The listing builds one solid part. Answer for the finished solid, in the listing's coordinates (mm). Face numbers are marked on the shaded views. Round coordinates to 2 decimals unless told otherwise and drop trailing zeros. Write each loop counter-clockwise with the first axis right and the second up, starting at its lowest first coordinate (ties: lowest second). Pieces come first, ordered by that corner, then holes. Notation, with made-up numbers: (-20.75, -10.75) - (-3.75, -10.75) arc R26 ccw to (-3.75, 11.25) - close; hole circle Ø11 at (-20, -37.5). An arc over 180 degrees is marked (long way). Use a Markdown table: item, result. Add a question column.
1) A cutting plane is placed at C-C (y = 24.5). Give the vertices of the cut face in (x, z) (3 decimals).
2) Each of these flat-tipped pins is pushed along its axis until it touches: P1, Ø5, axis at y = 7, z = 12.5, coming from the -X side; P2, Ø4.5, axis at x = -33.23, y = -33.23, coming from the -Z side; P3, Ø3, axis at x = -1.5, y = 22.5, coming from the +Z side; P4, Ø1.5, axis at x = -4, z = 3.5, coming from the +Y side. Where does it stop, or does it pass through?
3) A cutting plane is placed at A-A (z = 2.25). State how many separate pieces and enclosed holes the cut face has, then the cut area to 3 significant figures.
4) A cutting plane is placed at D-D (z = 9.75). Give the vertices of the cut face in (x, y), then the cut area to 3 significant figures.
5) Determine the mould class of the marked faces 1, 2, 3 and 4 for opening direction Y: +Y half, -Y half, draft (parallel to the pull), parting line (faces both ways), or undercut.
6) Find the intervals of material crossed by probe 1 along Y at (x, z) = (0, 21); probe 2 along Y at (x, z) = (-3, 18); probe 3 along Y at (x, z) = (-1, 10), in increasing order. Write a range as from..to.
7) A cutting plane is placed at B-B (x = -7.5). Give the vertices of the cut face in (y, z), then the cut area to 3 significant figures.
```python
from build123d import *

# Parameters (mm, degrees)
SKETCH1_R                       = 35
SKETCH1_R_2                     = 26
BOSS_EXTRUDE1_DEPTH             = 5
F_3_0MM_DOWEL_HOLE1_D           = 3
F_3_0MM_DOWEL_HOLE1_CSINK_D     = 3.05
F_3_0MM_DOWEL_HOLE1_CSINK_ANGLE = 90
SKETCH5_R                       = 40
SKETCH5_R_2                     = 35
BOSS_EXTRUDE2_DEPTH             = 22
BOSS_EXTRUDE3_START             = -5
SKETCH6_R                       = 52
SKETCH6_R_2                     = 35
BOSS_EXTRUDE3_DEPTH             = 5
F_4_0MM_DOWEL_HOLE2_D           = 4
F_4_0MM_DOWEL_HOLE2_CSINK_D     = 4.05
F_4_0MM_DOWEL_HOLE2_CSINK_ANGLE = 90
CUT_EXTRUDE1_DEPTH              = 3


with BuildPart() as part:
    # Sketch1 → Boss-Extrude1 (new body)
    with BuildSketch(Plane.XY):
        Circle(SKETCH1_R)
        Circle(SKETCH1_R_2, mode=Mode.SUBTRACT)
    extrude(amount=BOSS_EXTRUDE1_DEPTH)

    # Ø3.0mm Dowel Hole1 (through all)
    with Locations(Plane(origin=(0, 0, 0), x_dir=(-1, 0, 0), z_dir=(0, 0, -1))):
        with Locations((21.213203436, 21.213203436), (0, 30), (-21.213203436, 21.213203436), (-30, 0), (-21.213203436, -21.213203436), (0, -30), (21.213203436, -21.213203436), (30, 0)):
            CounterSinkHole(F_3_0MM_DOWEL_HOLE1_D / 2, F_3_0MM_DOWEL_HOLE1_CSINK_D / 2, counter_sink_angle=F_3_0MM_DOWEL_HOLE1_CSINK_ANGLE)

    # Sketch5 → Boss-Extrude2 (add)
    with BuildSketch(Plane(origin=(0, 0, 0), x_dir=(-1, 0, 0), z_dir=(0, 0, -1))):
        Circle(SKETCH5_R)
        Circle(SKETCH5_R_2, mode=Mode.SUBTRACT)
    extrude(amount=-BOSS_EXTRUDE2_DEPTH)

    # Sketch6 → Boss-Extrude3 (add)
    with BuildSketch(Plane.XY.offset(22).offset(BOSS_EXTRUDE3_START)):
        Circle(SKETCH6_R)
        with Locations(Location((0, 0, 0), (0, 0, 180))):
            Circle(SKETCH6_R_2, mode=Mode.SUBTRACT)
    extrude(amount=BOSS_EXTRUDE3_DEPTH)

    # Ø4.0mm Dowel Hole2 (through all)
    with Locations(Plane.XY.offset(22)):
        with Locations((0, 47), (-33.234018716, 33.234018716), (-47, 0), (-33.234018716, -33.234018716), (0, -47), (33.234018716, -33.234018716), (47, 0), (33.234018716, 33.234018716)):
            CounterSinkHole(F_4_0MM_DOWEL_HOLE2_D / 2, F_4_0MM_DOWEL_HOLE2_CSINK_D / 2, counter_sink_angle=F_4_0MM_DOWEL_HOLE2_CSINK_ANGLE)

    # Sketch10 → Cut-Extrude1 (cut)
    with BuildSketch(Plane(origin=(0, 0, 17), x_dir=(-1, 0, 0), z_dir=(0, 0, -1))):
        Polygon((36.500005039, 29.968032392), (37.695439002, 34.429452679), (34.429452679, 37.695439002), (29.968032392, 36.500005039), (28.772598429, 32.038584753), (32.038584753, 28.772598429), align=None)
        Polygon((4.618802154, 47), (2.309401077, 51), (-2.309401077, 51), (-4.618802154, 47), (-2.309401077, 43), (2.309401077, 43), align=None)
        Polygon((47, -4.618802154), (51, -2.309401077), (51, 2.309401077), (47, 4.618802154), (43, 2.309401077), (43, -2.309401077), align=None)
        Polygon((29.968032392, -36.500005039), (34.429452679, -37.695439002), (37.695439002, -34.429452679), (36.500005039, -29.968032392), (32.038584753, -28.772598429), (28.772598429, -32.038584753), align=None)
        Polygon((-4.618802154, -47), (-2.309401077, -51), (2.309401077, -51), (4.618802154, -47), (2.309401077, -43), (-2.309401077, -43), align=None)
        Polygon((-36.500005039, -29.968032392), (-37.695439002, -34.429452679), (-34.429452679, -37.695439002), (-29.968032392, -36.500005039), (-28.772598429, -32.038584753), (-32.038584753, -28.772598429), align=None)
        Polygon((-47, 4.618802154), (-51, 2.309401077), (-51, -2.309401077), (-47, -4.618802154), (-43, -2.309401077), (-43, 2.309401077), align=None)
        Polygon((-29.968032392, 36.500005039), (-34.429452679, 37.695439002), (-37.695439002, 34.429452679), (-36.500005039, 29.968032392), (-32.038584753, 28.772598429), (-28.772598429, 32.038584753), align=None)
    extrude(amount=-CUT_EXTRUDE1_DEPTH, mode=Mode.SUBTRACT)


solid = part.part
```
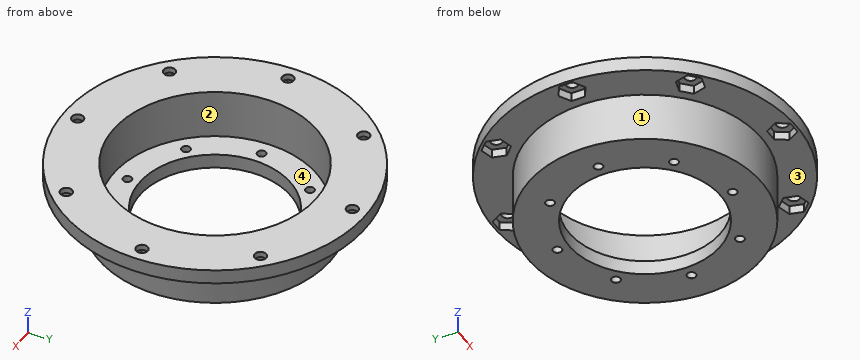
Entries:
| question | item | result |
|---|---|---|
| 1 | outline | (-45.867, 17) - (-31.619, 17) - (-31.619, 0) - (-8.703, 0) - (-8.703, 5) - (-24.995, 5) - (-24.995, 22) - (-45.867, 22) - close; (8.703, 0) - (31.619, 0) - (31.619, 17) - (45.867, 17) - (45.867, 22) - (24.995, 22) - (24.995, 5) - (8.703, 5) - close |
| 2 | P1 | stops at x = -39.75 |
| 2 | P2 | stops at z = 20 |
| 2 | P3 | passes through |
| 2 | P4 | stops at y = 39.87 |
| 3 | separate pieces | 1 |
| 3 | enclosed holes | 9 |
| 3 | area | 2,850 mm² |
| 4 | outline | circle Ø80 at (0, 0); hole circle Ø70 at (0, 0) |
| 4 | area | 1,180 mm² |
| 5 | face 1 | parting line |
| 5 | face 2 | undercut |
| 5 | face 3 | draft |
| 5 | face 4 | undercut |
| 6 | probe 1 | y = -52..-49, -45..-35, 35..45, 49..52 |
| 6 | probe 2 | y = -51.91..-49.8, -44.2..-34.87, 34.87..44.2, 49.8..51.91 |
| 6 | probe 3 | y = -39.99..-34.99, 34.99..39.99 |
| 7 | outline | (-51.46, 17) - (-39.29, 17) - (-39.29, 0) - (-24.89, 0) - (-24.89, 5) - (-34.19, 5) - (-34.19, 22) - (-51.46, 22) - close; (24.89, 0) - (39.29, 0) - (39.29, 17) - (51.46, 17) - (51.46, 22) - (34.19, 22) - (34.19, 5) - (24.89, 5) - close |
| 7 | area | 439 mm² |
